Autodesk Inventor part; units mm, degrees
ref_plane "YZ Plane" through (0, 0, 0) normal (1, 0, 0) x (0, 1, 0)
ref_plane "XZ Plane" through (0, 0, 0) normal (0, 1, 0) x (-1, 0, 0)
ref_plane "XY Plane" through (0, 0, 0) normal (0, 0, 1) x (1, 0, 0)
sketch "Эскиз1" plane through (0, 0, 0) normal (0, 0, 1) x (1, 0, 0)
  line L0 (0, -300) -> (18, -300)
  line L1 (18, 300) -> (0, 300)
  line L2 (0, 300) -> (0, -300)
  arc A0 (336.2347, 208.6518) -> (18, 300) centre (18, -300) ccw
  line L3 (18, -300) -> (336.2347, 208.6518)
  point P0 (0, 0)
  dimension "d0" = 600
  dimension "d1" = 18
  dimension "d5" = 18
extrude "Выдавливание1" add sketch "Эскиз1" along normal mid plane 32
properties part number "Веер хвоста (сложенный)"
Design review of the part built by this model. Coordinates are the model's own, in mm. Give positions to 0.01 mm unless a question says otherwise; leave off trailing zeros. Loops run counter-clockwise (first coordinate to the right, second up) from the corner with the lowest first, then second, coordinate; pieces in that order, holes last. Notation, with made-up numbers: M 50,2 L 74,2 A14 ccw 74,19 Z; hole C -21,36 d11. An arc over 180 degrees is marked long. Return JSON: item names as keys, results as strings. Group by question number.
Item 1: We need section C-C (x = 64). Give the boundary of the cut face in (y, z).
Item 2: We need section A-A (z = 0). Give the boundary of the cut face in (x, y), and give its area (3 significant figures).
Item 3: We need section B-B (y = 263). Give the boundary of the cut face in (x, z), and give its area (3 significant figures).
Item 4: Insertion check: pin 1 Ø1.5 at (y, z) = (113, -2) entering from +X; pin 2 Ø12 at (y, z) = (-214, -4) entering from +X; pin 3 Ø2 at (y, z) = (140, -10.5) entering from +X. Each pin has a flat end and moves straight along its axis. Give the tip position at first contact, or say it passes through.
Item 5: For probe 1 along X at (y, z) = (136.5, 0); probe 2 along X at (y, z) = (-124, -0.5); probe 3 along Y at (x, z) = (127.5, -7), list the stretches that pass through material, from the lowest coordinate up.
Output:
{
 "1": {"outline": "M -226.48,-16 L 298.23,-16 L 298.23,16 L -226.48,16 Z"},
 "2": {"outline": "M 0,-300 L 18,-300 L 336.23,208.65 A600 ccw 18,300 L 0,300 Z", "area": "111,000 mm^2"},
 "3": {"outline": "M 0,-16 L 225.44,-16 L 225.44,16 L 0,16 Z", "area": "7,210 mm^2"},
 "4": {"pin 1": "stops at x = 276.86", "pin 2": "stops at x = 75.56", "pin 3": "stops at x = 293.91"},
 "5": {"probe 1": "x = 0 to 291.09", "probe 2": "x = 0 to 128.11", "probe 3": "y = -124.98 to 289.92"}
}
